```python
from build123d import *

# Parameters (mm, degrees)
BOSS_EXTRUDE1_DEPTH = 12.5
SKETCH3_R           = 6.3525
CUT_EXTRUDE1_DEPTH  = 9.7
FILLET1_R           = 2
CUT_EXTRUDE2_DEPTH  = 9.7
FILLET2_R           = 2
SKETCH7_W           = 21
SKETCH7_H           = 7.555
CUT_EXTRUDE3_DEPTH  = 8
FILLET3_R           = 2
CHAMFER1_SIZE       = 0.25


with BuildPart() as part:
    # Sketch2 → Boss-Extrude1 (new body, symmetric)
    with BuildSketch(Plane.XY):
        with BuildLine():
            Line((3.125, 22.23), (3.125, 39.905))
            Line((3.125, 39.905), (5, 39.905))
            Line((5, 39.905), (5, -3.35))
            Line((5, -3.35), (-5, -3.35))
            Line((-5, -3.35), (-5, 17.905))
            Line((-5, 17.905), (-1.2, 17.905))
            ThreePointArc((-1.2, 17.905), (1.858236829, 19.171763171), (3.125, 22.23))
        make_face()
    extrude(amount=BOSS_EXTRUDE1_DEPTH, both=True)

    # Sketch3 → Cut-Extrude1 (cut)
    with BuildSketch(Plane.XZ.offset(3.35)):
        Circle(SKETCH3_R)
    extrude(amount=-CUT_EXTRUDE1_DEPTH, mode=Mode.SUBTRACT)

    # Fillet1
    fillet1_edges = [part.edges().sort_by_distance(p)[0] for p in [
        (4.0625, 39.905, 12.5),
        (4.0625, 39.905, -12.5),
    ]]
    fillet(fillet1_edges, radius=FILLET1_R)

    # Sketch6 → Cut-Extrude2 (cut)
    with BuildSketch(Plane.XZ.offset(3.35)):
        Polygon((0, 24.544175246), (-5.421515272, 4.310804798), (-5.421515272, 3.310804798), (-5.421515272, 0), (-10.421515272, 0), (-10.421515272, 29.544175246), (10.421515272, 29.544175246), (10.421515272, 0), (5.421515272, 0), (5.421515272, 3.310804798), (5.421515272, 4.310804798), align=None)
    cut_extrude2 = extrude(amount=-CUT_EXTRUDE2_DEPTH, mode=Mode.SUBTRACT)

    # Mirror1: Cut-Extrude2 across plane
    add(cut_extrude2.mirror(Plane.XY), mode=Mode.SUBTRACT)

    # Fillet2
    fillet2_edges = [part.edges().sort_by_distance(p)[0] for p in [
        (-3.227227031, 1.5, 12.5),
        (3.227227031, 1.5, 12.5),
        (5, 1.5, 5.883921208),
        (-5, 1.5, 5.883921208),
        (-3.227227031, 1.5, -12.5),
        (3.227227031, 1.5, -12.5),
        (-5, 1.5, -5.883921208),
        (5, 1.5, -5.883921208),
    ]]
    fillet(fillet2_edges, radius=FILLET2_R)

    # Sketch7 → Cut-Extrude3 (cut)
    with BuildSketch(Plane.ZY.offset(5)):
        with Locations((0, 12.1275)):
            Rectangle(SKETCH7_W, SKETCH7_H)
    extrude(amount=-CUT_EXTRUDE3_DEPTH, mode=Mode.SUBTRACT)

    # Fillet3
    fillet3_edges = [part.edges().sort_by_distance(p)[0] for p in [
        (-1, 8.35, -10.5),
        (-1, 15.905, -10.5),
        (-1, 15.905, 10.5),
        (-1, 8.35, 10.5),
    ]]
    fillet(fillet3_edges, radius=FILLET3_R)

    # Chamfer1
    chamfer1_edges = [part.edges().sort_by_distance(p)[0] for p in [
        (-5, 12.1275, 10.5),
        (-5, 8.35, 0),
        (-5, 12.1275, -10.5),
        (-5, 15.905, 0),
        (-5, 8.935786438, 9.914213562),
        (-5, 8.935786438, -9.914213562),
        (-5, 15.319213562, 9.914213562),
        (-5, 15.319213562, -9.914213562),
        (3.125, 39.905, 0),
        (3.125, 30.0675, -12.5),
        (3.125, 30.0675, 12.5),
        (3.125, 39.319213562, 11.914213562),
        (1.858236829, 19.171763171, 12.5),
        (3.125, 39.319213562, -11.914213562),
        (-3.1, 17.905, 12.5),
        (-3.1, 17.905, -12.5),
        (1.858236829, 19.171763171, -12.5),
    ]]
    chamfer(chamfer1_edges, length=CHAMFER1_SIZE)


solid = part.part
```
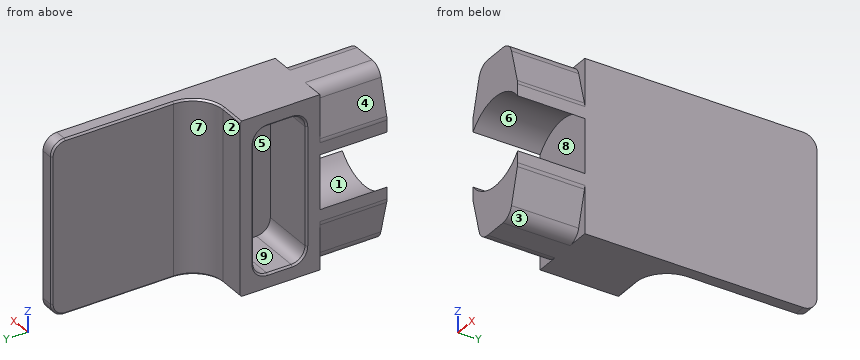
The listing builds one solid part. Answer for the finished solid, in the listing's coordinates (mm). Face numbers are marked on the shaded views. A direction names the side the tool comes from. Coordinates: 2 decimals unless noted, no trailing zeros. Write each loop counter-clockwise with the first axis right and the second up, starting at its lowest first coordinate (ties: lowest second). Pieces come first, ordered by that corner, then holes.
Q1. The mould has two halves that part along Y. Classify the marked faces 6, 7, 8 and 9: released by +Y, released by -Y, zero draft, split by the parting line, or undercut.
Returned:
face 6: zero draft
face 7: released by +Y
face 8: released by -Y
face 9: undercut
Q2. Section A-A, the plane y = 5 is taken. Write down the section's boundary in (x, z) (1 decimal).
Returned:
outline: (-5, -5.6) arc R2 ccw to (-4.9, -6.1) - (-3.6, -11) arc R2 ccw to (-1.7, -12.5) - (1.7, -12.5) arc R2 ccw to (3.6, -11) - (4.9, -6.1) arc R2 ccw to (5, -5.6) - (5, -3.9) arc R6.4 cw to (-5, -3.9) - close; (-5, 3.9) arc R6.4 cw to (5, 3.9) - (5, 5.6) arc R2 ccw to (4.9, 6.1) - (3.6, 11) arc R2 ccw to (1.7, 12.5) - (-1.7, 12.5) arc R2 ccw to (-3.6, 11) - (-4.9, 6.1) arc R2 ccw to (-5, 5.6) - close
Q3. Find the intervals of material crossed by line 1 along Y through (x, z) = (-1.5, -1.75) (3 decimals); line 2 along Z through (x, y) = (0.25, 1); line 3 along Y through (x, z) = (4, 0) (3 decimals), in increasing order.
Returned:
line 1: y = 6.35 to 8.35, 15.905 to 17.905
line 2: z = -12.5 to -6.35, 6.35 to 12.5
line 3: y = 6.35 to 39.905
Q4. Section D-D, the plane y = 29 is taken. Write down the section's boundary in (x, z) (3 decimals).
Returned:
outline: (3.125, -12.25) - (3.375, -12.5) - (5, -12.5) - (5, 12.5) - (3.375, 12.5) - (3.125, 12.25) - close
Q5. Section B-B, the plane z = -1.5 is taken. Write down the section's boundary in (x, y) (3 decimals), then the cut area to 3 significant figures.
Returned:
outline: (-5, 6.35) - (5, 6.35) - (5, 39.905) - (3.375, 39.905) - (3.125, 39.655) - (3.125, 22.23) arc R4.325 cw to (-1.2, 17.905) - (-5, 17.905) - (-5, 16.155) - (-4.75, 15.905) - (3, 15.905) - (3, 8.35) - (-4.75, 8.35) - (-5, 8.1) - close
area: 100 mm2
Q6. Section C-C, the plane x = -2.25 is taken. Write down the section's boundary in (y, z) (3 decimals), then the cut area to 3 significant figures.
Returned:
outline: (-3.35, -12.421) - (6.35, -12.421) - (6.35, -12.5) - (17.655, -12.5) - (17.905, -12.25) - (17.905, 12.25) - (17.655, 12.5) - (6.35, 12.5) - (6.35, 12.421) - (-3.35, 12.421) - (-3.35, 5.941) - (6.35, 5.941) - (6.35, -5.941) - (-3.35, -5.941) - close; hole (8.35, -8.5) arc R2 ccw to (10.35, -10.5) - (13.905, -10.5) arc R2 ccw to (15.905, -8.5) - (15.905, 8.5) arc R2 ccw to (13.905, 10.5) - (10.35, 10.5) arc R2 ccw to (8.35, 8.5) - close
area: 259 mm2
Q7. Which of the six approach directions +Z, -Z, +X, -X, +Y, -Y give full straight-line access (tool end or side, diameter ignored) to the marked faces 1, 2, 3, 4 and 5?
Returned:
face 1: -Y
face 2: +Z, -Z, -X, +Y
face 3: -Z, +X, -Y
face 4: +Z, -X, -Y
face 5: -X
Q8. Given P1, Ø1.1, axis at x = -4, z = 3, coming from the +Y side (3 decimals); P2, Ø4, axis at x = -2, z = 1, coming from the +Y side; P3, Ø6, axis at x = 2, y = 32.5, coming from the -Z side; P4, Ø4, axis at y = 11.5, z = 5, coming from the -X side, each flat-ended and moving along its own axis, determine where each tip first touches the part or whether it passes through.
Returned:
P1: stops at y = 17.905
P2: stops at y = 18.07
P3: stops at z = -12.5
P4: stops at x = 3
